Geometry check sheet. Reference: the model listing, model coordinates, mm. A direction names the side the tool comes from. Coordinates: 2 decimals unless noted, no trailing zeros.
Autodesk Inventor part; units mm, degrees
ref_plane "YZ Plane" through (0, 0, 0) normal (1, 0, 0) x (0, 1, 0)
ref_plane "XZ Plane" through (0, 0, 0) normal (0, 1, 0) x (-1, 0, 0)
ref_plane "XY Plane" through (0, 0, 0) normal (0, 0, 1) x (1, 0, 0)
sketch "Sketch1" plane through (0, 0, 0) normal (0, 0, 1) x (1, 0, 0)
  line L0 (0, 0) -> (25, 600)
  line L1 (25, 600) -> (375, 600)
  line L2 (375, 600) -> (400, 0)
  line L3 (400, 0) -> (0, 0)
  line L4 (0, 0) -> (76.2678, 0) construction
  line L5 (76.2678, 0) -> (120.3096, 19.0389) construction
  line L6 (120.3096, 19.0389) -> (188.6298, 38.3438) construction
  line L7 (188.6298, 38.3438) -> (327.7567, 0) construction
  line L8 (327.7567, 0) -> (400, 0) construction
  spline S0 degree 4 poles (0, 0) (76.2678, 0) (120.3096, 19.0389) (188.6298, 38.3438) (327.7567, 0) (400, 0) knots 1 1 1 1 1 2 3 3 3 3 3
  arc A0 (120.3096, 600) -> (279.6904, 600) centre (200, 673.1568) ccw
  line L9 (120.3096, 600) -> (25, 600)
  line L10 (25, 600) -> (0, 0)
  dimension "d0" = 600
  dimension "d1" = 25
  dimension "d2" = 350
  dimension "d3" = 400
  dimension "d4" = 175
extrude "Extrusion1" add sketch "Sketch1" along normal blind 50 contours L0 L1 A0 L2 S0
fillet "Fillet1" radius 20 9 edges at (327.3452, 600, 0) (387.5, 300, 0) (200, 564.9788, 0) (72.6548, 600, 0) (12.5, 300, 0) (25, 600, 25) (120.3096, 600, 25) (279.6904, 600, 25) (375, 600, 25)
fillet "Fillet2" radius 5 9 edges at (78.071, 600, 50) (119.3501, 598.5837, 50) (200, 564.9788, 50) (280.6499, 598.5837, 50) (321.929, 600, 50) (369.6606, 594.4335, 50) (387.8993, 290.4163, 50) (12.1007, 290.4163, 50) (30.3394, 594.4335, 50)
properties part number "backrest wheelchair EG26"
1. Gauge pin test, flat ends, axial feed: pin 1 Ø1.5 at (y, z) = (221, 8.5) entering from -X; pin 2 Ø10 at (y, z) = (485, 42) entering from -X; pin 3 Ø10 at (y, z) = (63.5, 9) entering from -X. Record the tip position at first contact, or that the pin passes through.
Computed values:
pin 1: stops at x = 12.34
pin 2: stops at x = 20
pin 3: stops at x = 3.55
2. Thickness scan on line 1 along Y through (x, z) = (277, 34); line 2 along Y through (x, z) = (80, 43); line 3 along X through (y, z) = (31.5, 20.5). Record the ranges inside material, lowest first.
Computed values:
line 1: y = 12.85 to 596.68
line 2: y = 6.03 to 600
line 3: x = 1.31 to 398.69
3. Draft check along Z on faces 3 (the cylindrical face through (18.28, 294.23, 5.7)), 4 (the flat face through (387.73, 294.48, 32.33)), 5 (the cylindrical face through (386.64, 286.29, 48.5)). Enter one of: released by +Z, released by -Z, zero draft, split by the parting line, or undercut.
Computed values:
face 3: released by -Z
face 4: zero draft
face 5: released by +Z
4. Access from +Z, -Z, +X, -X, +Y, -Y to the whole of each face (thin tool, end or side, straight path). Record for faces 1 (the cylindrical face through (13.695, 294.423, 48.496)), 2 (the cylindrical face through (119.449, 598.544, 32.675)).
Computed values:
face 1: +Z, -X, +Y
face 2: +Z, -Z, +Y
